Check sheet for the modelled part. Datum: model origin and axes. Units: mm. Face numbers are marked on the shaded views. A direction names the side the tool comes from. Give positions to 0.01 mm unless a question says otherwise; leave off trailing zeros. Order: outer loops, then holes, each group sorted by start corner. A loop starts at its lowest first (then second) coordinate and runs counter-clockwise, first axis right, second up. Notation, with made-up numbers: (-21.75, 15.25) -> (26.25, 15.25) arc R36 ccw to (26.25, 51.25) -> close; hole circle Ø3 at (45.5, 73). An arc over 180 degrees is marked (long way). Answer in a Markdown table with one row per item. Add a question column.
(1) Go/stop test with flat-tipped pins: pin 1 (1.6 mm diameter, centred on y = -20.5, z = 8, fed in from -X); pin 2 (3.5 mm diameter, centred on x = 5, z = 16.4, fed in from +Y); pin 3 (3.5 mm diameter, centred on x = 29.3, z = 17.4, fed in from -Y). Record where each tip stops, or that it passes through.
(2) Cross-section at B-B (y = -30.5). Record the cut outline in (x, z), then the cut area to 3 significant figures.
(3) Cross-section at D-D (z = 8). Record the cut outline in (x, y).
(4) Cross-section at C-C (x = 5). Record the cut outline in (y, z).
(5) Release check for a two-part mould opening along Z. For the marked faces 1, 2 and 3 record: released by +Z, released by -Z, zero draft, split by the parting line, or undercut.
(6) Thickness scan on L1, parallel to X at y = -21.5, z = 13.75; L2, parallel to Y at x = 3, z = 18.5; L3, parallel to X at y = -30.7, z = 16.4. Record the ranges inside material, lowest first. Write a range as [from, to].
(7) Cross-section at A-A (x = 29.3). Record the cut outline in (y, z).
(8) Set-up check for the marked faces 4, 5, 6 and 7: record each of +Z, -Z, +X, -X, +Y, -Y from which the full face is reachable in a straight line by a thin tool's end or side.
```python
from build123d import *

# Parameters (mm, degrees)
SKETCH_1_W          = 42
SKETCH_1_H          = 21.4
EXTRUDE_1_DEPTH     = 12
SKETCH_2_W          = 6
SKETCH_2_H          = 2
CUT_EXTRUDE_1_DEPTH = 49.641134855
SKETCH_3_R          = 3.1
CUT_EXTRUDE_2_DEPTH = 2.6
SKETCH_4_R          = 2.25
CUT_EXTRUDE_3_DEPTH = 10
SKETCH_4_3_R        = 1.5
CUT_EXTRUDE_4_DEPTH = 49.641134855
SKETCH_5_W          = 88.870895105
SKETCH_5_H          = 42.258480341
CUT_EXTRUDE_5_DEPTH = 53.01884274


with BuildPart() as part:
    # 草图1 → 凸台-拉伸1 (new body)
    with BuildSketch(Plane(origin=(0, 0, 0), x_dir=(1, 0, 0), z_dir=(0, 1, 0))):
        with Locations((21, -10.7)):
            Rectangle(SKETCH_1_W, SKETCH_1_H)
    extrude(amount=EXTRUDE_1_DEPTH)

    # 草图2 → 切除-拉伸1 (cut, through all)
    with BuildSketch(Plane(origin=(0, 0, 0), x_dir=(-1, 0, 0), z_dir=(0, 0, -1))):
        Polygon((-10, 0), (0, 0), (0, 10), (-10, 10), (-10, 2), align=None)
        with Locations((-13, 1)):
            Rectangle(SKETCH_2_W, SKETCH_2_H)
    extrude(amount=-CUT_EXTRUDE_1_DEPTH, mode=Mode.SUBTRACT)

    # 草图3 → 切除-拉伸2 (cut)
    with BuildSketch(Plane.XZ):
        with Locations(Location((20.3, 14, 0), (0, 0, 270))):
            Circle(SKETCH_3_R)
    extrude(amount=-CUT_EXTRUDE_2_DEPTH, mode=Mode.SUBTRACT)

    # 草图4 → 切除-拉伸3 (cut)
    with BuildSketch(Plane(origin=(0, 12, 0), x_dir=(1, 0, 0), z_dir=(0, 1, 0))):
        with Locations(Location((29.3, -17.4, 0), (0, 0, 270))):
            Circle(SKETCH_4_R)
        with Locations(Location((38, -8, 0), (0, 0, 270))):
            Circle(SKETCH_4_R)
    extrude(amount=-CUT_EXTRUDE_3_DEPTH, mode=Mode.SUBTRACT)

    # 草图4<3> → 切除-拉伸4 (cut, through all)
    with BuildSketch(Plane(origin=(0, 12, 0), x_dir=(1, 0, 0), z_dir=(0, 1, 0))):
        with Locations(Location((5, -5, 0), (0, 0, 270))):
            Circle(SKETCH_4_3_R)
        with Locations(Location((5, -16.4, 0), (0, 0, 270))):
            Circle(SKETCH_4_3_R)
        with Locations(Location((38, -8, 0), (0, 0, 270))):
            Circle(SKETCH_4_3_R)
        with Locations(Location((29.3, -17.4, 0), (0, 0, 270))):
            Circle(SKETCH_4_3_R)
    extrude(amount=-CUT_EXTRUDE_4_DEPTH, mode=Mode.SUBTRACT)


with BuildPart() as body_2:
    # 镜向1: mirrored copy
    add(part.part.mirror(Plane.ZX.offset(-10)))


with BuildPart() as part_1:
    add(part.part)

    # 草图5 → 切除-拉伸5 (cut, through all)
    with BuildSketch(Plane(origin=(0, -10, 0), x_dir=(1, 0, 0), z_dir=(0, 1, 0))):
        with Locations((22.816673382, -12.28482211)):
            Rectangle(SKETCH_5_W, SKETCH_5_H)
    extrude(amount=CUT_EXTRUDE_5_DEPTH, mode=Mode.SUBTRACT)


solid = body_2.part
```
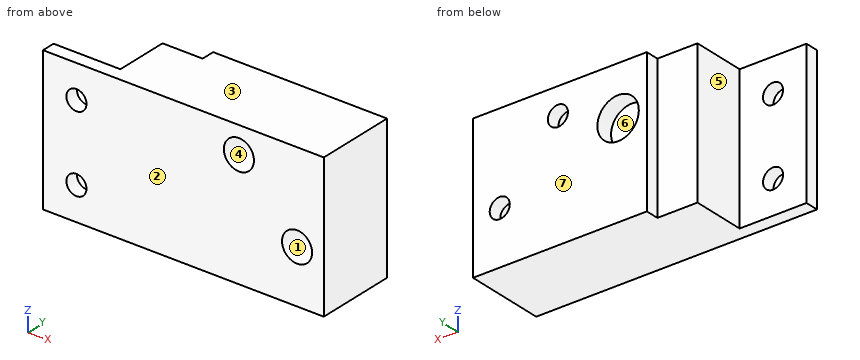
Answer below:
| question | item | result |
|---|---|---|
| 1 | pin 1 | stops at x = 16 |
| 1 | pin 2 | stops at y = -30 |
| 1 | pin 3 | stops at y = -22 |
| 2 | outline | (0, 0) -> (42, 0) -> (42, 21.4) -> (0, 21.4) -> close; hole circle Ø3 at (5, 5); hole circle Ø3 at (5, 16.4); hole circle Ø4.5 at (29.3, 17.4); hole circle Ø4.5 at (38, 8) |
| 2 | area | 853 mm² |
| 3 | outline | (0, -32) -> (35.75, -32) -> (35.75, -22) -> (36.5, -22) -> (36.5, -20) -> (16, -20) -> (16, -22) -> (10, -22) -> (10, -30) -> (0, -30) -> close; (39.5, -22) -> (40.25, -22) -> (40.25, -32) -> (42, -32) -> (42, -20) -> (39.5, -20) -> close |
| 4 | outline | (-32, 0) -> (-30, 0) -> (-30, 3.5) -> (-32, 3.5) -> close; (-32, 6.5) -> (-30, 6.5) -> (-30, 14.9) -> (-32, 14.9) -> close; (-32, 17.9) -> (-30, 17.9) -> (-30, 21.4) -> (-32, 21.4) -> close |
| 5 | face 1 | undercut |
| 5 | face 2 | zero draft |
| 5 | face 3 | released by +Z |
| 6 | L1 | x = [16, 17.21], [23.39, 42] |
| 6 | L2 | y = [-32, -30] |
| 6 | L3 | x = [0, 3.5], [6.5, 27.28], [31.32, 42] |
| 7 | outline | (-32, 0) -> (-20, 0) -> (-20, 15.9) -> (-22, 15.9) -> (-22, 15.15) -> (-32, 15.15) -> close; (-32, 19.65) -> (-22, 19.65) -> (-22, 18.9) -> (-20, 18.9) -> (-20, 21.4) -> (-32, 21.4) -> close |
| 8 | face 4 | -Y |
| 8 | face 5 | +Z, -Z, -X, +Y |
| 8 | face 6 | +Y |
| 8 | face 7 | +Z, -Z, +X, -X, +Y |
